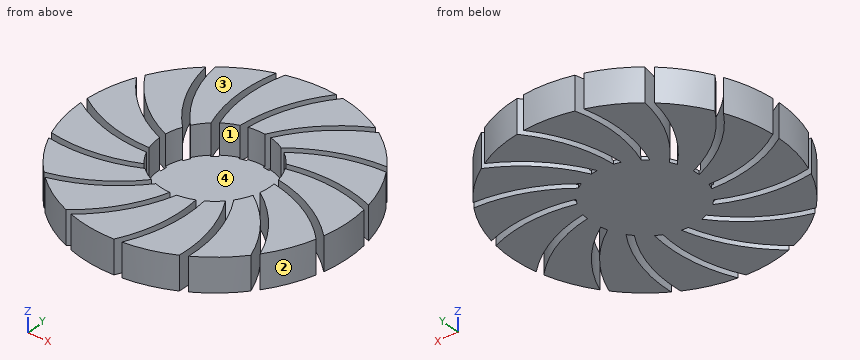
from build123d import *

# Parameters (mm, degrees)
SKETCH_R           = 40
PAD_DEPTH          = 10
POCKET_DEPTH       = 237.157334
POLARPATTERN_COUNT = 15
SKETCH002_R        = 16.5
POCKET001_DEPTH    = 9


with BuildPart() as part:
    # Sketch → Pad (new body)
    with BuildSketch(Plane.XY):
        Circle(SKETCH_R)
    extrude(amount=PAD_DEPTH)

    # Sketch001 (on Face1 of ShapeBinder) → Pocket (cut, through all)
    with BuildSketch(Plane.XY.offset(10)):
        with BuildLine():
            ThreePointArc((-36.92851, 17.8125), (-27.922716, 7.192654), (-16, 0))
            Line((-15.874508, 2), (-16, 0))
            ThreePointArc((-35.895192, 19.8125), (-27.374199, 9.232269), (-15.874508, 2))
            Line((-35.895192, 19.8125), (-36.92851, 17.8125))
        make_face()
    pocket = extrude(amount=-POCKET_DEPTH, mode=Mode.SUBTRACT)

    # PolarPattern: Pocket ×15 about axis
    polarpattern_axis = Axis((0, 0, 0), (0, 0, 1))
    for i in range(1, POLARPATTERN_COUNT):
        add(pocket.rotate(polarpattern_axis, i * 360 / POLARPATTERN_COUNT), mode=Mode.SUBTRACT)

    # Sketch002 (on Face4 of PolarPattern) → Pocket001 (cut)
    with BuildSketch(Plane.XY.offset(10)):
        Circle(SKETCH002_R)
    extrude(amount=-POCKET001_DEPTH, mode=Mode.SUBTRACT)


with BuildPart() as part_1:
    # Body placement: moved
    add(part.part.moved(Location((50, 63, 63))))


solid = part_1.part
Model file for the job. Use its own axes, mm. Face numbers are marked on the shaded views. Coordinates: 2 decimals unless noted, no trailing zeros. Write each loop counter-clockwise with the first axis right and the second up, starting at its lowest first coordinate (ties: lowest second). Pieces come first, ordered by that corner, then holes. Notation, with made-up numbers: (75, -5) -> (90, -5) arc R16 cw to (90, 15) -> close; hole circle Ø6 at (47, 24.5). An arc over 180 degrees is marked (long way). One line per item, written item: value. Start each with the question number.
1) Flat gauge pins, fed straight in: pin 1 Ø6 at (x, z) = (43, 64.5) entering from -Y; pin 2 Ø2 at (y, z) = (70, 68.5) entering from -X; pin 3 Ø2 at (x, z) = (60.5, 67.5) entering from -Y. Where does each tip first touch, or does it go through?
2) Probe probe 1 along Y at (x, z) = (14, 64); probe 2 along Y at (x, z) = (79, 71.75); probe 3 along X at (y, z) = (92, 67.5). List the from-to ranges inside material, lowest first.
3) Pull direction Y, two halves, no side cores. Call the marked faces 1, 2, 3 and 4: +Y half, -Y half, draft (parallel to the pull), parting line (faces both ways), or undercut.
4) Slice it at C-C on y = 44. Write the cut outline in (x, z).
5) Slice it at D-D on x = 77.5. Write the cut outline in (y, z).
6) Slice it at B-B on x = 32. Write the cut outline in (y, z).
7) Slice it at A-A on x = 20. Write the cut outline in (y, z), then the cut area to 3 significant figures.
Answers follow:
1. pin 1: y = 23.2
1. pin 2: x = 10.45
1. pin 3: y = 24.14
2. probe 1: 45.56 to 47.14, 49.06 to 61.24, 63.39 to 79.34
2. probe 2: 35.45 to 41.29, 45.4 to 59.49, 61.67 to 71.45, 73.37 to 83.79, 85.71 to 90.55
2. probe 3: 22.45 to 23.85, 25.78 to 36.7, 38.6 to 48.3, 50.37 to 62.3, 65.39 to 77.55
3. face 1: undercut
3. face 2: -Y half
3. face 3: draft
3. face 4: undercut
4. outline: (14.8, 63) -> (38.65, 63) -> (38.65, 73) -> (14.8, 73) -> close; (41.5, 63) -> (48.64, 63) -> (48.64, 73) -> (41.5, 73) -> close; (50.67, 63) -> (56.53, 63) -> (56.53, 73) -> (50.67, 73) -> close; (58.43, 63) -> (65.44, 63) -> (65.44, 73) -> (58.43, 73) -> close; (67.45, 63) -> (77.61, 63) -> (77.61, 73) -> (67.45, 73) -> close; (79.77, 63) -> (85.2, 63) -> (85.2, 73) -> (79.77, 73) -> close
5. outline: (33.95, 63) -> (44.2, 63) -> (44.2, 73) -> (33.95, 73) -> close; (47.82, 63) -> (60.32, 63) -> (60.32, 73) -> (47.82, 73) -> close; (62.45, 63) -> (71.63, 63) -> (71.63, 73) -> (62.45, 73) -> close; (73.54, 63) -> (83.56, 63) -> (83.56, 73) -> (73.54, 73) -> close; (85.49, 63) -> (92.05, 63) -> (92.05, 73) -> (85.49, 73) -> close
6. outline: (27.28, 63) -> (37.23, 63) -> (37.23, 73) -> (27.28, 73) -> close; (39.38, 63) -> (48.31, 63) -> (48.31, 73) -> (39.38, 73) -> close; (50.29, 63) -> (56.5, 63) -> (56.5, 73) -> (50.29, 73) -> close; (58.4, 63) -> (63.86, 63) -> (63.86, 73) -> (58.4, 73) -> close; (65.96, 63) -> (73.43, 63) -> (73.43, 73) -> (65.96, 73) -> close; (76.7, 63) -> (98.72, 63) -> (98.72, 73) -> (76.7, 73) -> close
7. outline: (36.54, 63) -> (46.68, 63) -> (46.68, 73) -> (36.54, 73) -> close; (48.58, 63) -> (58.71, 63) -> (58.71, 73) -> (48.58, 73) -> close; (60.72, 63) -> (72.08, 63) -> (72.08, 73) -> (60.72, 73) -> close; (74.79, 63) -> (89.46, 63) -> (89.46, 73) -> (74.79, 73) -> close
7. area: 463 mm2
